Model file for the job. Use its own axes, mm. A direction names the side the tool comes from. Round coordinates to 2 decimals unless told otherwise and drop trailing zeros. Loops run counter-clockwise (first coordinate to the right, second up) from the corner with the lowest first, then second, coordinate; pieces in that order, holes last. Notation, with made-up numbers: (11.5, -1.75) -> (53.5, -1.75) arc R17 cw to (53.5, 9.25) -> close; hole circle Ø11 at (61, 62.5). An arc over 180 degrees is marked (long way). Use a Markdown table: item, result.
from build123d import *

# Parameters (mm, degrees)
F0_R     = 6.5
F1_DEPTH = 20
F2_SIZE  = 5
F3_W     = 30
F3_H     = 30
F4_DEPTH = 1
F6_DEPTH = 25


with BuildPart() as f1:
    # F0 (on Front) → F1 (new body)
    with BuildSketch(Plane.XZ):
        Circle(F0_R)
    extrude(amount=F1_DEPTH)

    # F2
    f2_edges = [f1.edges().sort_by_distance(p)[0] for p in [
        (-6.5, -20, 0),
    ]]
    chamfer(f2_edges, length=F2_SIZE)

    # F3 (on Front) → F4 (join)
    with BuildSketch(Plane.XZ):
        Rectangle(F3_W, F3_H)
    extrude(amount=F4_DEPTH)

    # F5 (on Front) → F6 (cut)
    with BuildSketch(Plane.XZ):
        with BuildLine():
            Line((-1.5, 0), (-7.5, 0))
            ThreePointArc((-7.5, 0), (-5.303301, -5.303301), (0, -7.5))
            Line((0, -7.5), (0, -1.5))
            ThreePointArc((0, -1.5), (1.06066, -1.06066), (1.5, 0))
            Line((1.5, 0), (7.5, 0))
            ThreePointArc((7.5, 0), (5.303301, 5.303301), (0, 7.5))
            Line((0, 7.5), (0, 1.5))
            ThreePointArc((0, 1.5), (-1.06066, 1.06066), (-1.5, 0))
        make_face()
    extrude(amount=F6_DEPTH, mode=Mode.SUBTRACT)


solid = f1.part
Q1. Band-saw the part on D-D, the plane x = 8.25. Give the cut face in (y, z), plus the area to 3 significant figures.
Results list:
| item | result |
|---|---|
| outline | (-1, -15) -> (0, -15) -> (0, 15) -> (-1, 15) -> close |
| area | 30.0 mm² |
Q2. Band-saw the part on C-C, the plane z = 11.5. Give the cut face in (x, y).
Results list:
| item | result |
|---|---|
| outline | (-15, -1) -> (15, -1) -> (15, 0) -> (-15, 0) -> close |
Q3. Pull direction Z, two halves, no side cores. Call faces 4 (the face through (15, -0.5, -0.2)), 5 (the face through (-5.361, -0.493, -5.245)), 6 (the face through (-2.77, -17.54, 2.83)): released by +Z, released by -Z, zero draft, split by the parting line, or undercut.
Results list:
| item | result |
|---|---|
| face 4 | zero draft |
| face 5 | undercut |
| face 6 | released by +Z |
Q4. Flat gauge pins, fed straight in: pin 1 (4 mm diameter, centred on x = 0.5, z = -3.5, fed in from -Y); pin 2 (8 mm diameter, centred on x = 5, z = -2.5, fed in from -Y); pin 3 (8 mm diameter, centred on x = 7, z = 9, fed in from -Y). Where does each tip first touch, or does it go through?
Results list:
| item | result |
|---|---|
| pin 1 | stops at y = -19.96 |
| pin 2 | stops at y = -19.91 |
| pin 3 | stops at y = -1 |
Q5. Band-saw the part on A-A, the plane y = -18. Give the cut face in (x, z), plus the area to 3 significant figures.
Results list:
| item | result |
|---|---|
| outline | (-3.5, 0) -> (-1.5, 0) arc R1.5 cw to (0, 1.5) -> (0, 3.5) arc R3.5 ccw to start; (0, -3.5) arc R3.5 ccw to (3.5, 0) -> (1.5, 0) arc R1.5 cw to (0, -1.5) -> close |
| area | 15.7 mm² |
Q6. Band-saw the part on B-B, the plane y = -9.25. Give the cut face in (x, z), plus the area to 3 significant figures.
Results list:
| item | result |
|---|---|
| outline | (-6.5, 0) -> (-1.5, 0) arc R1.5 cw to (0, 1.5) -> (0, 6.5) arc R6.5 ccw to start; (0, -6.5) arc R6.5 ccw to (6.5, 0) -> (1.5, 0) arc R1.5 cw to (0, -1.5) -> close |
| area | 62.8 mm² |
Q7. Tool access for faces 1 (the face through (-6.9, -1, 0.2)), 2 (the face through (4.545, -7.902, -4.646)), 3 (the face through (0, -8, -4)): list every direction of +Z, -Z, +X, -X, +Y, -Y with a clear straight run to the whole face (end or side of a thin tool).
Results list:
| item | result |
|---|---|
| face 1 | -Y |
| face 2 | -Z, +X, -Y |
| face 3 | +Y, -Y |
Q8. Drill centre lines: L1, parallel to Y at x = 10.5, z = -8.5; L2, parallel to X at y = -13, z = -3.5; L3, parallel to Z at x = 1, y = -3. Where is each one in solid material? Low to high. Write a range as from..to.
Results list:
| item | result |
|---|---|
| L1 | y = -1..0 |
| L2 | x = 0..5.48 |
| L3 | z = -6.42..-1.12 |
